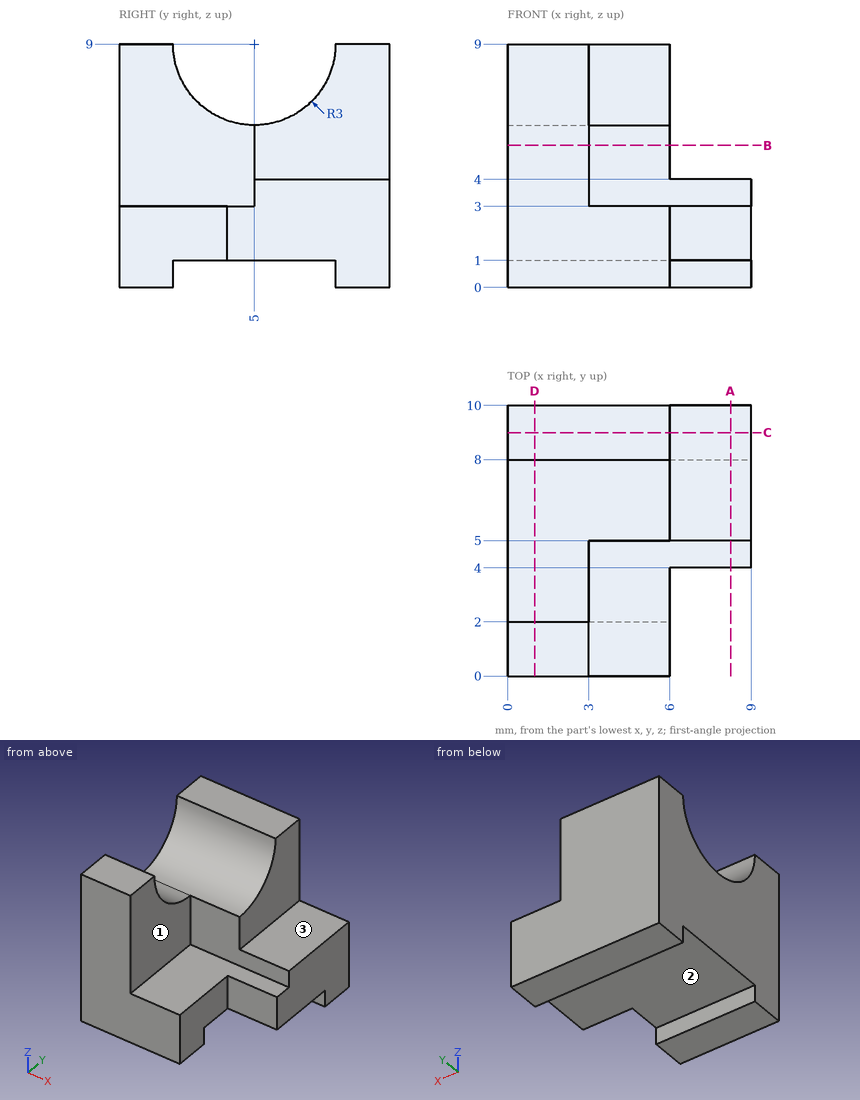
Geometry: see drawing. Coordinates: mm, zero at the bounding-box minimum. A direction names the side the tool comes from. Round coordinates to 2 decimals unless told otherwise and drop trailing zeros. Order: outer loops, then holes, each group sorted by start corner. A loop starts at its lowest first (then second) coordinate and runs counter-clockwise, first axis right, second up. Notation, with made-up numbers: (71.25, -12.75) -> (101.25, -12.75) arc R27 cw to (101.25, 15.25) -> close; hole circle Ø9 at (75, -6). An arc over 180 degrees is marked (long way). Write each question's results on one line, items separated by ' | '.
Q1. Section query A-A (x = 8.25). Output: boundary loops of the cut face in (y, z).
Response values:
outline: (4, 1) -> (8, 1) -> (8, 0) -> (10, 0) -> (10, 4) -> (5, 4) -> (5, 3) -> (4, 3) -> close
Q2. Ray query, line 1 along Y through (x, z) = (5, 0.75); line 2 along X through (y, z) = (8, 6.5); line 3 along X through (y, z) = (2.75, 3.25). Return the intervals inside material, ascending.
Response values:
line 1: 0 to 2, 8 to 10 | line 2: 0 to 6 | line 3: 0 to 3
Q3. Section query C-C (y = 9). Output: boundary loops of the cut face in (x, z), and give its area (3 significant figures).
Response values:
outline: (0, 0) -> (9, 0) -> (9, 4) -> (6, 4) -> (6, 9) -> (0, 9) -> close | area: 66.0 mm²
Q4. Section query D-D (x = 1). Output: boundary loops of the cut face in (y, z).
Response values:
outline: (0, 0) -> (2, 0) -> (2, 1) -> (8, 1) -> (8, 0) -> (10, 0) -> (10, 9) -> (8, 9) arc R3 cw to (2, 9) -> (0, 9) -> close
Q5. Access query for the marked faces 1, 2 and 3. Directions: +Z, -Z, +X, -X, +Y, -Y. A direction counts if a zero-diameter tool reaches every point of the face in a straight line with its end or side. Return the directions, or none.
Response values:
face 1: +Z, +X, -Y | face 2: -Z, +X, -X | face 3: +Z, +X, +Y, -Y
Q6. Pin query (flat end, axial travel): pin 1 Ø0.9 at (x, z) = (5, 5) entering from -Y; pin 2 Ø3 at (y, z) = (1, 3.5) entering from +X; pin 3 Ø0.9 at (x, y) = (7, 8.5) entering from +Z. Return the tip coordinate at first contact, or that it passes through.
Response values:
pin 1: y = 5 | pin 2: x = 6 | pin 3: z = 4
Q7. Section query B-B (z = 5.25). Output: boundary loops of the cut face in (x, y), and give its area (3 significant figures).
Response values:
outline: (0, 0) -> (3, 0) -> (3, 5) -> (6, 5) -> (6, 10) -> (0, 10) -> close | area: 45.0 mm²
